CAD build for the part. Positions are in the model's coordinates, mm. A direction names the side the tool comes from. Coordinates: 2 decimals unless noted, no trailing zeros. Loops run counter-clockwise (first coordinate to the right, second up) from the corner with the lowest first, then second, coordinate; pieces in that order, holes last. Notation, with made-up numbers: M -26,-4.5 L 11,-4.5 A34 ccw 11,30.5 Z; hole C 31,80 d3. An arc over 180 degrees is marked long. Answer as a JSON object with one key per item and string values. Group by question number.
```python
from build123d import *

# Parameters (mm, degrees)
F1_DEPTH = 63.5
F2_DEPTH = 25.4
F3_DEPTH = 7.9375
F5_R     = 5.08
F6_DEPTH = 25.4


with BuildPart() as f1:
    # F0 (on Front) → F1 (new body, symmetric)
    with BuildSketch(Plane.XZ):
        Polygon((-41.275, -9.525), (41.275, -9.525), (41.275, 9.525), (22.225, 9.525), (-41.275, 9.525), align=None)
    extrude(amount=F1_DEPTH, both=True)

    # F0 (on Front) → F2 (join, symmetric)
    with BuildSketch(Plane.XZ):
        with BuildLine():
            Line((22.225, 9.525), (41.275, 9.525))
            Line((41.275, 9.525), (41.275, 27.0002))
            ThreePointArc((41.275, 27.0002), (45.9246798487, 38.2255201513), (57.15, 42.8752))
            Line((57.15, 42.8752), (60.325, 42.8752))
            Line((60.325, 42.8752), (60.325, 61.9252))
            add(Edge.make_bspline(
                [(55.5200098819, 61.8871425031), (57.0859299245, 61.9054209742), (58.687127075, 61.9179033933), (60.325, 61.9252)],
                knots=[111.2130490849, 111.2130490849, 111.2130490849, 111.2130490849, 114.3168446032, 114.3168446032, 114.3168446032, 114.3168446032], degree=3))
            ThreePointArc((55.5200098819, 61.8871425031), (31.8845786709, 51.1127301464), (22.225, 27.0002))
            Line((22.225, 27.0002), (22.225, 9.525))
        make_face()
    extrude(amount=F2_DEPTH, both=True)

    # F0 (on Front) → F3 (join, symmetric)
    with BuildSketch(Plane.XZ):
        with BuildLine():
            add(Edge.make_bspline(
                [(-41.275, 9.525), (-11.4062497234, 53.1358095427), (-0.5889513978, 61.2322009997), (55.5200098819, 61.8871425031)],
                knots=[0, 0, 0, 0, 111.2130490849, 111.2130490849, 111.2130490849, 111.2130490849], degree=3))
            Line((-41.275, 9.525), (22.225, 9.525))
            Line((22.225, 9.525), (22.225, 27.0002))
            ThreePointArc((22.225, 27.0002), (31.8845786709, 51.1127301464), (55.5200098819, 61.8871425031))
        make_face()
    extrude(amount=F3_DEPTH, both=True)

    # F0 (on Front) → F4 (revolve)
    with BuildSketch(Plane.XZ):
        Polygon((85.725, 66.675), (85.725, 61.9252), (85.725, 42.8752), (85.725, 38.1), (111.125, 38.1), (111.125, 66.675), align=None)
    revolve(axis=Axis((85.725, 0, 52.3875), (0, 0, 1)))

    # F5
    f5_edges = [f1.edges().sort_by_distance(p)[0] for p in [
        (-41.275, -63.5, 0),
        (41.275, -63.5, 0),
        (-41.275, 63.5, 0),
        (41.275, 63.5, 0),
    ]]
    fillet(f5_edges, radius=F5_R)

    # F6 (add): faces of the model
    f6_faces = [f1.faces().sort_by_distance(p)[0] for p in [
        (60.325, 12.7, 52.4002),
        (60.325, -12.7, 52.4002),
    ]]
    extrude(f6_faces, amount=F6_DEPTH)


solid = f1.part
```
Item 1: Tool access for faces 4 (the flat face through (65, 19, 61.925)), 5 (the cylindrical face through (32.14, -16.79, 51.38)), 6 (the flat face through (46, 25.4, 41)): list every direction of +Z, -Z, +X, -X, +Y, -Y with a clear straight run to the whole face (end or side of a thin tool).
Item 2: Drill centre lines: L1, parallel to Y at x = 73, z = 54.5; L2, parallel to Z at x = -5, y = 28.5 (3 decimals); L3, parallel to Y at x = 31.5, z = 58. Where is each one in solid material? Low to high. Write a range as from..to.
Item 3: Pull direction X, two halves, no side cores. Call faces 1 (the flat face through (22.225, -17, 18)), 2 (the flat face through (1, 35, 9.525)), 3 (the cylindrical face through (45.8, -0.4, 38.1)): released by +X, released by -X, zero draft, split by the parting line, or undercut.
Item 4: Slice it at A-A, the plane z = 2. Write the cut outline in (x, y) (3 decimals).
Item 5: Pin check, flat tips, straight feed: pin 1 (2 mm diameter, centred on y = -38.5, z = 4, fed in from +X) (3 decimals); pin 2 (8.5 mm diameter, centred on y = -15.5, z = 21.5, fed in from -X) (3 decimals); pin 3 (1.5 mm diameter, centred on x = 53, z = 42.5, fed in from -Y). Stop position of each tip, or through.
Item 6: Slice it at B-B, the plane y = -30.5. Write the cut outline in (x, z) (3 decimals).
Computed:
{
 "1": {"face 4": "+Z, -X, +Y", "face 5": "+Z, -X, -Y", "face 6": "+Z, +X, -X, +Y"},
 "2": {"L1": "-25.4..25.4", "L2": "-9.525..9.525", "L3": "-7.94..7.94"},
 "3": {"face 1": "released by -X", "face 2": "zero draft", "face 3": "undercut"},
 "4": {"outline": "M -41.275,-58.42 A5.08 ccw -36.195,-63.5 L 36.195,-63.5 A5.08 ccw 41.275,-58.42 L 41.275,58.42 A5.08 ccw 36.195,63.5 L -36.195,63.5 A5.08 ccw -41.275,58.42 Z"},
 "5": {"pin 1": "x = 41.275", "pin 2": "x = 22.225", "pin 3": "y = -25.4"},
 "6": {"outline": "M -41.275,-9.525 L 41.275,-9.525 L 41.275,9.525 L -41.275,9.525 Z"}
}
